Geometry: final body of the model. Coordinates: model frame, mm. Face numbers are marked on the shaded views. A direction names the side the tool comes from. Give positions to 0.01 mm unless a question says otherwise; leave off trailing zeros. Write each loop counter-clockwise with the first axis right and the second up, starting at its lowest first coordinate (ties: lowest second). Pieces come first, ordered by that corner, then holes. Notation, with made-up numbers: (47, 73.25) -> (55, 73.25) arc R10 cw to (55, 82.25) -> close; hole circle Ø6 at (0.25, -20). An arc over 180 degrees is marked (long way). Answer as a JSON object with one key per item and string values.
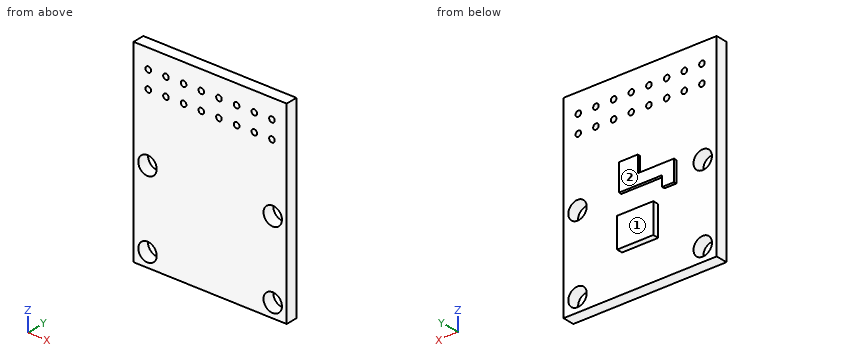
from build123d import *

# Parameters (mm, degrees)
BOSS_EXTRUDE1_DEPTH = 0.85
SKETCH2_R           = 1.325
SKETCH2_R_2         = 0.4
CUT_EXTRUDE1_DEPTH  = 2.7
SKETCH3_W           = 5.2
SKETCH3_H           = 4.3
BOSS_EXTRUDE2_DEPTH = 0.85
BOSS_EXTRUDE3_DEPTH = 0.4


with BuildPart() as part:
    # Sketch1 → Boss-Extrude1 (new body, symmetric)
    with BuildSketch(Plane(origin=(0, 0, 0), x_dir=(1, 0, 0), z_dir=(0, 1, 0))):
        Polygon((-11, -7.5), (-11, -20.5), (11, -20.5), (11, -7.5), (11, 7.5), (-11, 7.5), align=None)
    extrude(amount=BOSS_EXTRUDE1_DEPTH, both=True)

    # Sketch2 → Cut-Extrude1 (cut, through all)
    with BuildSketch(Plane(origin=(0, 0.85, 0), x_dir=(1, 0, 0), z_dir=(0, 1, 0))):
        with Locations((-9, 5.5)):
            Circle(SKETCH2_R)
        with Locations((9, 5.5)):
            Circle(SKETCH2_R)
        with Locations((9, -5.5)):
            Circle(SKETCH2_R)
        with Locations((-9, -5.5)):
            Circle(SKETCH2_R)
        with Locations((-8.89, -15.19)):
            Circle(SKETCH2_R_2)
        with Locations((-6.35, -15.19)):
            Circle(SKETCH2_R_2)
        with Locations((-3.81, -15.19)):
            Circle(SKETCH2_R_2)
        with Locations((-1.27, -15.19)):
            Circle(SKETCH2_R_2)
        with Locations((1.27, -15.19)):
            Circle(SKETCH2_R_2)
        with Locations((3.81, -15.19)):
            Circle(SKETCH2_R_2)
        with Locations((6.35, -15.19)):
            Circle(SKETCH2_R_2)
        with Locations((8.89, -15.19)):
            Circle(SKETCH2_R_2)
        with Locations((-6.35, -17.73)):
            Circle(SKETCH2_R_2)
        with Locations((-3.81, -17.73)):
            Circle(SKETCH2_R_2)
        with Locations((-1.27, -17.73)):
            Circle(SKETCH2_R_2)
        with Locations((1.27, -17.73)):
            Circle(SKETCH2_R_2)
        with Locations((3.81, -17.73)):
            Circle(SKETCH2_R_2)
        with Locations((6.35, -17.73)):
            Circle(SKETCH2_R_2)
        with Locations((8.89, -17.73)):
            Circle(SKETCH2_R_2)
        with Locations((-8.89, -17.73)):
            Circle(SKETCH2_R_2)
    extrude(amount=-CUT_EXTRUDE1_DEPTH, mode=Mode.SUBTRACT)

    # Sketch3 → Boss-Extrude2 (add)
    with BuildSketch(Plane(origin=(0, 0.85, 0), x_dir=(1, 0, 0), z_dir=(0, 1, 0))):
        Rectangle(SKETCH3_W, SKETCH3_H)
    extrude(amount=BOSS_EXTRUDE2_DEPTH)

    # Sketch3<3> → Boss-Extrude3 (add)
    with BuildSketch(Plane(origin=(0, 0.85, 0), x_dir=(1, 0, 0), z_dir=(0, 1, 0))):
        Polygon((-5.2, -3.825), (-5.2, -6.825), (0, -6.825), (0, -9.2), (2.7, -9.2), (2.7, -5.325), (-3.5, -5.325), (-3.5, -3.825), align=None)
    extrude(amount=BOSS_EXTRUDE3_DEPTH)


solid = part.part
Q1. Cut plane B-B (x = -1.27). Return the cut outline in (y, z) (3 decimals).
Values:
{"outline": "(-0.85, -7.5) -> (0.85, -7.5) -> (0.85, -2.15) -> (1.7, -2.15) -> (1.7, 2.15) -> (0.85, 2.15) -> (0.85, 5.325) -> (1.25, 5.325) -> (1.25, 6.825) -> (0.85, 6.825) -> (0.85, 14.79) -> (-0.85, 14.79) -> close; (-0.85, 15.59) -> (0.85, 15.59) -> (0.85, 17.33) -> (-0.85, 17.33) -> close; (-0.85, 18.13) -> (0.85, 18.13) -> (0.85, 20.5) -> (-0.85, 20.5) -> close"}
Q2. Cut plane A-A (z = -5.5). Return the cut outline in (x, y) (3 decimals), and give its area (3 significant figures).
Values:
{"outline": "(-11, -0.85) -> (-10.325, -0.85) -> (-10.325, 0.85) -> (-11, 0.85) -> close; (-7.675, -0.85) -> (7.675, -0.85) -> (7.675, 0.85) -> (-7.675, 0.85) -> close; (10.325, -0.85) -> (11, -0.85) -> (11, 0.85) -> (10.325, 0.85) -> close", "area": "28.4 mm²"}
Q3. Cut plane C-C (y = -0.25). State how many separate pieces and enclosed holes the cut face has, and give its area (3 significant figures).
Values:
{"separate pieces": "1", "enclosed holes": "20", "area": "586 mm²"}
Q4. Cut plane D-D (x = -9). Return the cut outline in (y, z) (3 decimals).
Values:
{"outline": "(-0.85, -7.5) -> (0.85, -7.5) -> (0.85, -6.825) -> (-0.85, -6.825) -> close; (-0.85, -4.175) -> (0.85, -4.175) -> (0.85, 4.175) -> (-0.85, 4.175) -> close; (-0.85, 6.825) -> (0.85, 6.825) -> (0.85, 14.805) -> (-0.85, 14.805) -> close; (-0.85, 15.575) -> (0.85, 15.575) -> (0.85, 17.345) -> (-0.85, 17.345) -> close; (-0.85, 18.115) -> (0.85, 18.115) -> (0.85, 20.5) -> (-0.85, 20.5) -> close"}
Q5. Material intervals for L1, parallel to Z at x = -3.81, y = 0.3; L2, parallel to X at y = 0.15, z = -5.5 (3 decimals); L3, parallel to Z at x = 9.75, y = -0.5, sorted ascending. Write a range as from..to.
Values:
{"L1": "-7.5..14.79, 15.59..17.33, 18.13..20.5", "L2": "-11..-10.325, -7.675..7.675, 10.325..11", "L3": "-7.5..-6.59, -4.41..4.41, 6.59..20.5"}
Q6. First-contact query: P1, Ø0.7, axis at x = 1, y = 1, coming from the +Z side; P2, Ø0.7, axis at y = 1.5, z = 1, coming from the -X side; P3, Ø4.5, axis at x = 0.5, z = 6, coming from the +Y side; P4, Ø1.6, axis at x = -9, z = -5.5, coming from the +Y side. Flat tips, straight axial feed; report the tip coordinate or a pass-through.
Values:
{"P1": "z = 20.5", "P2": "x = -2.6", "P3": "y = 1.25", "P4": "through"}
Q7. Set-up query: the marked faces 1 and 2. Return all of +Z, -Z, +X, -X, +Y, -Y with unobstructed straight access to the full face (end or side cutting, diameter ignored); none if empty.
Values:
{"face 1": "+Z, -Z, +X, -X, +Y", "face 2": "+Z, +X, -X, +Y"}
